Work out the finished part from the listing and answer in its coordinate system (mm). Round coordinates to 2 decimals unless told otherwise and drop trailing zeros. Loops run counter-clockwise (first coordinate to the right, second up) from the corner with the lowest first, then second, coordinate; pieces in that order, holes last.
```python
from build123d import *

# Parameters (mm, degrees)
SKETCH_1_R      = 4
SKETCH_1_R_2    = 25
EXTRUDE_1_DEPTH = 15


with BuildPart() as part:
    # 草图1 → 凸台-拉伸1 (new body)
    with BuildSketch(Plane.XY):
        Polygon((-46.25, 38.25), (-21.25, 38.25), (130.53, 38.25), (133.03, 38.25), (133.03, -38.25), (130.53, -38.25), (-21.25, -38.25), (-46.25, -38.25), (-48.75, -38.25), (-48.75, 38.25), align=None)
        with Locations((-33.75, 26.25)):
            Circle(SKETCH_1_R, mode=Mode.SUBTRACT)
        with Locations(Location((-33.75, -26.25, 0), (0, 0, 180))):
            Circle(SKETCH_1_R, mode=Mode.SUBTRACT)
        with Locations((118.03, 19)):
            Circle(SKETCH_1_R, mode=Mode.SUBTRACT)
        with Locations(Location((118.03, -19, 0), (0, 0, 180))):
            Circle(SKETCH_1_R, mode=Mode.SUBTRACT)
        with Locations((6.75, 0)):
            Circle(SKETCH_1_R_2, mode=Mode.SUBTRACT)
    extrude(amount=EXTRUDE_1_DEPTH)


solid = part.part
```
1. Find section A-A (x = 6.75). Write down the section's boundary in (y, z).
Answer key:
outline: (-38.25, 0) - (-25, 0) - (-25, 15) - (-38.25, 15) - close; (25, 0) - (38.25, 0) - (38.25, 15) - (25, 15) - close
2. Consider probe 1 along Y at (x, z) = (-33.75, 5.75); probe 2 along Y at (x, z) = (6.75, 4); probe 3 along Y at (x, z) = (119, 13.5). Determine where each line is inside the solid, lowest interval first.
Answer key:
probe 1: y = -38.25 to -30.25, -22.25 to 22.25, 30.25 to 38.25
probe 2: y = -38.25 to -25, 25 to 38.25
probe 3: y = -38.25 to -22.88, -15.12 to 15.12, 22.88 to 38.25
3. Find section D-D (y = 2). Write down the section's boundary in (x, z), then the cut area to 3 significant figures.
Answer key:
outline: (-48.75, 0) - (-18.17, 0) - (-18.17, 15) - (-48.75, 15) - close; (31.67, 0) - (133.03, 0) - (133.03, 15) - (31.67, 15) - close
area: 1,980 mm2
4. Find section B-B (x = -33.75). Write down the section's boundary in (y, z), then the cut area to 4 significant figures.
Answer key:
outline: (-38.25, 0) - (-30.25, 0) - (-30.25, 15) - (-38.25, 15) - close; (-22.25, 0) - (22.25, 0) - (22.25, 15) - (-22.25, 15) - close; (30.25, 0) - (38.25, 0) - (38.25, 15) - (30.25, 15) - close
area: 907.5 mm2
5. Determine the mould class of faces 1 (the face through (-48.75, -1, 7)), 2 (the face through (114.034, 19.176, 7.395)), 3 (the face through (43, 38.25, 7)) for opening direction X: +X half, -X half, draft (parallel to the pull), parting line (faces both ways), or undercut.
Answer key:
face 1: -X half
face 2: undercut
face 3: draft
6. Given pin 1 (9 mm diameter, centred on x = 118.03, y = -19, fed in from +Z), flat-ended and moving along its own axis, determine where the tip first touches the part or whether it passes through.
Answer key:
pin 1: stops at z = 15
7. Find section C-C (z = 8.25). Write down the section's boundary in (x, y).
Answer key:
outline: (-48.75, -38.25) - (133.03, -38.25) - (133.03, 38.25) - (-48.75, 38.25) - close; hole circle Ø8 at (-33.75, -26.25); hole circle Ø8 at (-33.75, 26.25); hole circle Ø50 at (6.75, 0); hole circle Ø8 at (118.03, -19); hole circle Ø8 at (118.03, 19)
